Read the model definition and answer for the solid it produces. Units are mm, in the model's axes. Face numbers are marked on the shaded views. Round coordinates to 2 decimals unless told otherwise and drop trailing zeros. Write each loop counter-clockwise with the first axis right and the second up, starting at its lowest first coordinate (ties: lowest second). Pieces come first, ordered by that corner, then holes. Notation, with made-up numbers: (41, -24.75) - (66, -24.75) arc R30 ccw to (66, 1.25) - close; hole circle Ø8 at (11, 67.5). An arc over 180 degrees is marked (long way). One line per item, written item: value. Start each with the question number.
(1) The mould has two halves that part along Y. Classify the marked faces 1, 2, 3 and 4: +Y half, -Y half, draft (parallel to the pull), parting line (faces both ways), or undercut.
(2) A cutting plane is placed at C-C, the plane z = 1.9. Determine the outline of the cut face in (x, y), plus the area to 3 significant figures.
(3) A flat-ended cylindrical pin translates along its axis: pin 1 Ø18 at (x, y) = (0, 0) entering from -Z. Find the tip coordinate at first contact, or state that the pin passes through.
(4) Find the intervals of material crossed by L1, parallel to X at y = -11.25, z = 1.7; L2, parallel to Y at x = 0, z = 2.25; L3, parallel to Y at x = 11, z = 2.15, in increasing order.
(5) A cutting plane is placed at D-D, the plane y = -9.5. Determine the outline of the cut face in (x, z).
(6) A cutting plane is placed at A-A, the plane y = 0. Determine the outline of the cut face in (x, z).
from build123d import *

# Parameters (mm, degrees)
SKETCH1_W           = 30
SKETCH1_H           = 30
BOSS_EXTRUDE1_DEPTH = 3
SKETCH2_R           = 10
CUT_EXTRUDE1_DEPTH  = 3
SKETCH3_R           = 2.5
CUT_EXTRUDE2_DEPTH  = 10


with BuildPart() as part:
    # Sketch1 → Boss-Extrude1 (new body)
    with BuildSketch(Plane.XY):
        Rectangle(SKETCH1_W, SKETCH1_H)
    extrude(amount=BOSS_EXTRUDE1_DEPTH)

    # Sketch2 → Cut-Extrude1 (cut)
    with BuildSketch(Plane.XY.offset(3)):
        Circle(SKETCH2_R)
    extrude(amount=-CUT_EXTRUDE1_DEPTH, mode=Mode.SUBTRACT)

    # Sketch3 → Cut-Extrude2 (cut)
    with BuildSketch(Plane.XY.offset(3)):
        with Locations((-11.313708499, 11.313708499)):
            Circle(SKETCH3_R)
        with Locations((11.313708499, 11.313708499)):
            Circle(SKETCH3_R)
        with Locations((11.313708499, -11.313708499)):
            Circle(SKETCH3_R)
        with Locations((-11.313708499, -11.313708499)):
            Circle(SKETCH3_R)
    extrude(amount=-CUT_EXTRUDE2_DEPTH, mode=Mode.SUBTRACT)


solid = part.part
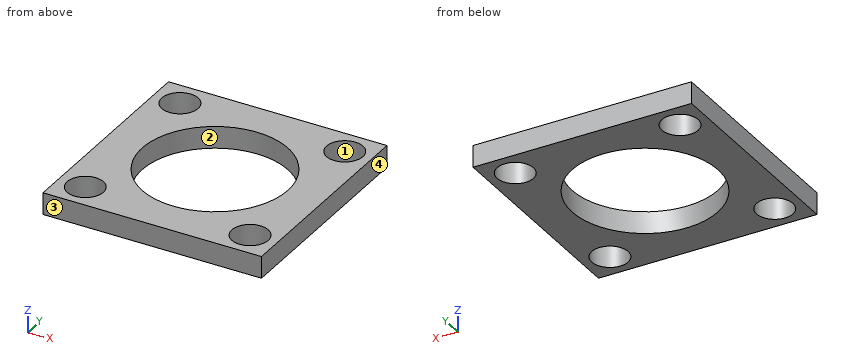
Here are the results:
1. face 1: undercut
1. face 2: undercut
1. face 3: -Y half
1. face 4: draft
2. outline: (-15, -15) - (15, -15) - (15, 15) - (-15, 15) - close; hole circle Ø5 at (-11.31, -11.31); hole circle Ø5 at (-11.31, 11.31); hole circle Ø20 at (0, 0); hole circle Ø5 at (11.31, -11.31); hole circle Ø5 at (11.31, 11.31)
2. area: 507 mm²
3. pin 1: through
4. L1: -15 to -13.81, -8.81 to 8.81, 13.81 to 15
4. L2: -15 to -10, 10 to 15
4. L3: -15 to -13.79, -8.83 to 8.83, 13.79 to 15
5. outline: (-15, 0) - (-13.03, 0) - (-13.03, 3) - (-15, 3) - close; (-9.59, 0) - (-3.12, 0) - (-3.12, 3) - (-9.59, 3) - close; (3.12, 0) - (9.59, 0) - (9.59, 3) - (3.12, 3) - close; (13.03, 0) - (15, 0) - (15, 3) - (13.03, 3) - close
6. outline: (-15, 0) - (-10, 0) - (-10, 3) - (-15, 3) - close; (10, 0) - (15, 0) - (15, 3) - (10, 3) - close
